For this review, take the finished solid that the model builds, in its own axes (mm). Round coordinates to 2 decimals unless told otherwise and drop trailing zeros. Order: outer loops, then holes, each group sorted by start corner. A loop starts at its lowest first (then second) coordinate and runs counter-clockwise, first axis right, second up. Notation, with made-up numbers: (10, 38.5) -> (64, 38.5) arc R22 cw to (64, 70.5) -> close; hole circle Ø6 at (15, 69). An arc over 180 degrees is marked (long way). Use a Markdown table: item, result. Add a question column.
1) Wall thickness on line 1 along Y through (x, z) = (0.4, 0); line 2 along Z through (x, y) = (-0.3, 105); line 3 along Y through (x, z) = (-2.5, -1.75): over which ranges is each line inside the solid? List them lowest first. Write a range as [from, to].
2) Consider section A-A (y = 95). State the section outline as (x, z) points.
3) Consider section C-C (x = 0). State the section outline as (y, z) points, plus the area to 3 significant figures.
4) Clearance check with flat-ended pins moving along their axes: P1, Ø2, axis at x = 0, y = 89, coming from the -Z side; P2, Ø1.4, axis at x = 0.5, y = 96, coming from the +Z side; P3, Ø1, axis at y = 71.5, z = 2.5, coming from the +X side; P4, Ø1.8, axis at y = 105, z = 0, coming from the +X side. State where each tip first meets the part, or that it passes through.
5) Consider section B-B (z = 0). State the section outline as (x, y) points.
```python
from build123d import *

# Parameters (mm, degrees)
SKETCH2_R           = 3.95
BOSS_EXTRUDE1_DEPTH = 80
SKETCH3_W           = 1.8
SKETCH3_H           = 3.8
BOSS_EXTRUDE3_DEPTH = 30
SKETCH5_R           = 1
CUT_EXTRUDE1_DEPTH  = 1.8


with BuildPart() as part:
    # Sketch2 → Boss-Extrude1 (new body)
    with BuildSketch(Plane(origin=(0, 0, 0), x_dir=(1, 0, 0), z_dir=(0, 1, 0))):
        with Locations(Location((0, 0, 0), (0, 0, 270))):  # turned: the seam where the file's is
            Circle(SKETCH2_R)
    extrude(amount=BOSS_EXTRUDE1_DEPTH)

    # Sketch3 → Boss-Extrude3 (add)
    with BuildSketch(Plane(origin=(0, 80, 0), x_dir=(1, 0, 0), z_dir=(0, 1, 0))):
        Rectangle(SKETCH3_W, SKETCH3_H)
    extrude(amount=BOSS_EXTRUDE3_DEPTH)

    # Sketch5 → Cut-Extrude1 (cut)
    with BuildSketch(Plane(origin=(0.9, 0, 0), x_dir=(0, 0, -1), z_dir=(1, 0, 0))):
        with Locations((0, 105)):
            Circle(SKETCH5_R)
        with Locations((0, 95)):
            Circle(SKETCH5_R)
    extrude(amount=-CUT_EXTRUDE1_DEPTH, mode=Mode.SUBTRACT)


solid = part.part
```
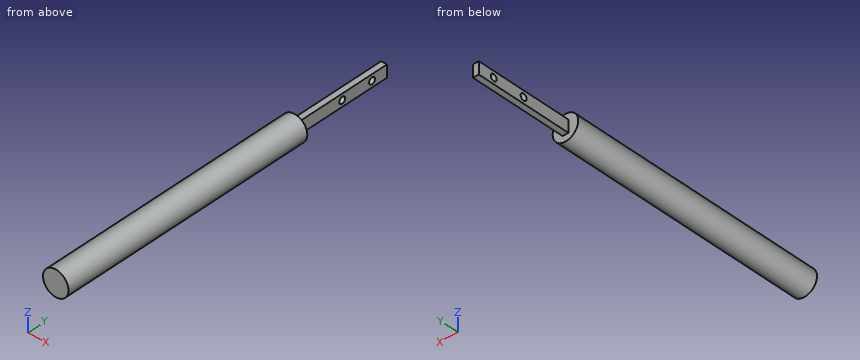
Results list:
| question | item | result |
|---|---|---|
| 1 | line 1 | [0, 94], [96, 104], [106, 110] |
| 1 | line 2 | [-1.9, -1], [1, 1.9] |
| 1 | line 3 | [0, 80] |
| 2 | outline | (-0.9, -1.9) -> (0.9, -1.9) -> (0.9, -1) -> (-0.9, -1) -> close; (-0.9, 1) -> (0.9, 1) -> (0.9, 1.9) -> (-0.9, 1.9) -> close |
| 3 | outline | (0, -3.95) -> (80, -3.95) -> (80, -1.9) -> (110, -1.9) -> (110, 1.9) -> (80, 1.9) -> (80, 3.95) -> (0, 3.95) -> close; hole circle Ø2 at (95, 0); hole circle Ø2 at (105, 0) |
| 3 | area | 740 mm2 |
| 4 | P1 | z = -1.9 |
| 4 | P2 | z = 1.9 |
| 4 | P3 | x = 3.41 |
| 4 | P4 | through |
| 5 | outline | (-3.95, 0) -> (3.95, 0) -> (3.95, 80) -> (0.9, 80) -> (0.9, 94) -> (-0.9, 94) -> (-0.9, 80) -> (-3.95, 80) -> close; (-0.9, 96) -> (0.9, 96) -> (0.9, 104) -> (-0.9, 104) -> close; (-0.9, 106) -> (0.9, 106) -> (0.9, 110) -> (-0.9, 110) -> close |
